Design review of the part built by this model. Coordinates are the model's own, in mm. Round coordinates to 2 decimals unless told otherwise and drop trailing zeros. Loops run counter-clockwise (first coordinate to the right, second up) from the corner with the lowest first, then second, coordinate; pieces in that order, holes last. Notation, with made-up numbers: M -36,-33.75 L 3,-33.75 A20 ccw 3,-18.75 Z; hole C 83.5,-9.75 d8. An arc over 180 degrees is marked long. Answer as CSV lines item,"result". Start each with the question number.
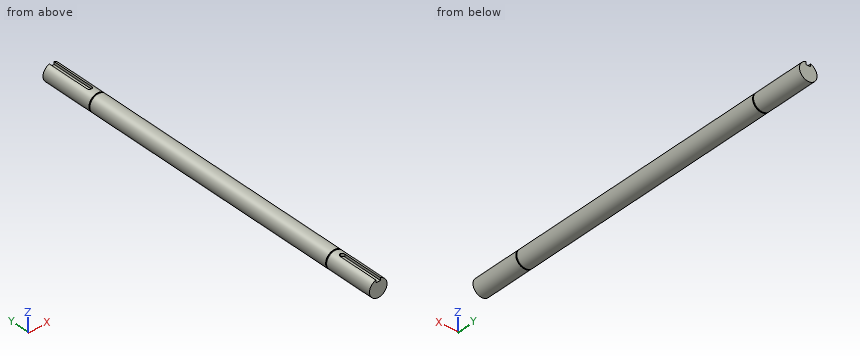
from build123d import *

# Parameters (mm, degrees)
F0_R      = 7.5
F1_DEPTH  = 320
F4_DEPTH  = 2.5
F6_R      = 7.5
F6_R_2    = 7
F7_DEPTH  = 1
F9_R      = 7.5
F9_R_2    = 7
F10_DEPTH = 1


with BuildPart() as f1:
    # F0 (on Front) → F1 (new body)
    with BuildSketch(Plane.XZ):
        Circle(F0_R)
    extrude(amount=F1_DEPTH)

    # F3 (on offset) → F4 (cut)
    with BuildSketch(Plane.XY.offset(7.5)):
        with BuildLine():
            Line((2, 0), (-2, 0))
            Line((-2, 0), (-2, -37))
            ThreePointArc((-2, -37), (-1.4142135624, -38.4142135624), (0, -39))
            ThreePointArc((0, -39), (1.4142135624, -38.4142135624), (2, -37))
            Line((2, -37), (2, 0))
        make_face()
        with BuildLine():
            Line((-2, -320), (2, -320))
            Line((2, -320), (2, -285))
            ThreePointArc((2, -285), (1.4142135624, -283.5857864376), (0, -283))
            ThreePointArc((0, -283), (-1.4142135624, -283.5857864376), (-2, -285))
            Line((-2, -285), (-2, -320))
        make_face()
    extrude(amount=-F4_DEPTH, mode=Mode.SUBTRACT)

    # F6 (on offset) → F7 (cut)
    with BuildSketch(Plane.XZ.offset(278)):
        Circle(F6_R)
        Circle(F6_R_2, mode=Mode.SUBTRACT)
    extrude(amount=-F7_DEPTH, mode=Mode.SUBTRACT)

    # F9 (on offset) → F10 (cut)
    with BuildSketch(Plane(origin=(0, -45, 0), x_dir=(-1, 0, 0), z_dir=(0, 1, 0))):
        Circle(F9_R)
        Circle(F9_R_2, mode=Mode.SUBTRACT)
    extrude(amount=-F10_DEPTH, mode=Mode.SUBTRACT)


solid = f1.part
Item 1: Insertion check: pin 1 Ø1.8 at (y, z) = (-306.5, 5.5) entering from +X; pin 2 Ø4.5 at (x, y) = (0.5, -11.5) entering from +Z; pin 3 Ø1.1 at (y, z) = (-26.5, 6) entering from -X. Each pin has a flat end and moves straight along its axis. Give the tip position at first contact, or say it passes through.
Item 2: To check wall thickness, follow line 1 (Y direction, x = -4.75, z = -5.25); line 2 (X direction, y = -176.5, z = -0.25); line 3 (Z direction, x = 0.5, y = -140). State the ranges of each line that lie inside material, in increasing order.
Item 3: Consider section A-A, the plane y = -205.5. Write out the cut boundary in (x, z), then the cut area to 3 significant figures.
Found:
1,pin 1,"stops at x = 5.92"
1,pin 2,"stops at z = 7.23"
1,pin 3,"stops at x = -5.15"
2,line 1,"y = -320 to -278, -277 to -46, -45 to 0"
2,line 2,"x = -7.5 to 7.5"
2,line 3,"z = -7.48 to 7.48"
3,outline,"C 0,0 d15"
3,area,"177 mm^2"
